The model under review builds one solid part; all positions refer to its coordinate system, in mm. A direction names the side the tool comes from. Coordinates: 2 decimals unless noted, no trailing zeros. Order: outer loops, then holes, each group sorted by start corner. A loop starts at its lowest first (then second) coordinate and runs counter-clockwise, first axis right, second up. Notation, with made-up numbers: (40.5, 25) -> (75.5, 25) arc R15 ccw to (75.5, 31) -> close; hole circle Ø2 at (38.5, 7.5). An arc over 180 degrees is marked (long way). Answer as CSV lines item,"result". Start each with the question number.
from build123d import *
from OCP.BRepFilletAPI import BRepFilletAPI_MakeFillet

# Parameters (mm, degrees)
CROQUIS2_W                 = 40
CROQUIS2_H                 = 15
SALIENTE_EXTRUIR1_DEPTH    = 65.5
REDONDEO1_R                = 1
CORTAR_EXTRUIR1_DEPTH      = 40
CORTAR_EXTRUIR4_DEPTH      = 1
CORTAR_EXTRUIR4_DEPTH_BACK = 10
CROQUIS9_W                 = 6
CROQUIS9_H                 = 15
CROQUIS10_W                = 6
CROQUIS10_H                = 15
CORTAR_EXTRUIR5_DEPTH      = 10
CROQUIS7_R                 = 2
CORTAR_EXTRUIR6_DEPTH      = 40
CROQUIS14_W                = 40.000001659
CROQUIS14_H                = 60.5
CORTAR_EXTRUIR9_DEPTH      = 2.6
REDONDEO5_R1               = 5
REDONDEO5_R2               = 1
CROQUIS16_W                = 32
CROQUIS16_H                = 4
CORTAR_EXTRUIR10_DEPTH     = 2.5


with BuildPart() as part:
    # Croquis2 → Saliente-Extruir1 (new body)
    with BuildSketch(Plane.XY):
        Rectangle(CROQUIS2_W, CROQUIS2_H)
    extrude(amount=SALIENTE_EXTRUIR1_DEPTH)

    # Redondeo1
    redondeo1_edges = [part.edges().sort_by_distance(p)[0] for p in [
        (-20, 0, 65.5),
        (0, -7.5, 65.5),
        (20, 0, 65.5),
        (0, -7.5, 0),
        (-20, 0, 0),
        (0, 7.5, 0),
        (20, 0, 0),
        (0, 7.5, 65.5),
        (20, -7.5, 32.75),
        (-20, -7.5, 32.75),
        (-20, 7.5, 32.75),
        (20, 7.5, 32.75),
    ]]
    fillet(redondeo1_edges, radius=REDONDEO1_R)

    # Croquis6 → Cortar-Extruir1 (cut)
    with BuildSketch(Plane(origin=(20, 0, 0), x_dir=(0, 0, -1), z_dir=(1, 0, 0))):
        Polygon((-60.5, 7.5), (-60.5, 0), (-55.501553512, 0), (-10, 0), (-10, 5), (-10, 7.5), align=None)
    extrude(amount=-CORTAR_EXTRUIR1_DEPTH, mode=Mode.SUBTRACT)

    # Croquis9 → Cortar-Extruir4 (cut, two sides: drawn at the far end of the back side and taken through both)
    with BuildSketch(Plane(origin=(0, 0, 0), x_dir=(-1, 0, 0), z_dir=(0, 0, -1)).offset(-CORTAR_EXTRUIR4_DEPTH_BACK)):
        with Locations((-17, 0)):
            Rectangle(CROQUIS9_W, CROQUIS9_H)
    extrude(amount=CORTAR_EXTRUIR4_DEPTH + CORTAR_EXTRUIR4_DEPTH_BACK, mode=Mode.SUBTRACT)

    # Croquis10 → Cortar-Extruir5 (cut)
    with BuildSketch(Plane(origin=(0, 0, 0), x_dir=(-1, 0, 0), z_dir=(0, 0, -1))):
        with Locations((17, 0)):
            Rectangle(CROQUIS10_W, CROQUIS10_H)
    extrude(amount=-CORTAR_EXTRUIR5_DEPTH, mode=Mode.SUBTRACT)

    # Croquis7 → Cortar-Extruir6 (cut)
    with BuildSketch(Plane(origin=(20, 0, 0), x_dir=(0, 0, -1), z_dir=(1, 0, 0))):
        with Locations((-5, 0)):
            Circle(CROQUIS7_R)
    extrude(amount=-CORTAR_EXTRUIR6_DEPTH, mode=Mode.SUBTRACT)

    # Croquis14 → Cortar-Extruir9 (cut)
    with BuildSketch(Plane(origin=(0, 7.5, 0), x_dir=(1, 0, 0), z_dir=(0, 1, 0))):
        with Locations((8.3e-07, -30.25)):
            Rectangle(CROQUIS14_W, CROQUIS14_H)
    extrude(amount=-CORTAR_EXTRUIR9_DEPTH, mode=Mode.SUBTRACT)

    # Redondeo5: one fillet with a radius per group of edges: ONE call of the kernel's fillet builder (fillet() takes one radius for all edges)
    redondeo5_edges_1 = [part.edges().sort_by_distance(p)[0] for p in [
        (0, 4.9, 0),
    ]]
    redondeo5_edges_2 = [part.edges().sort_by_distance(p)[0] for p in [
        (0, 4.9, 10),
    ]]
    redondeo5 = BRepFilletAPI_MakeFillet(part.part.solid().wrapped)
    for e in redondeo5_edges_1:
        redondeo5.Add(REDONDEO5_R1, e.wrapped)
    for e in redondeo5_edges_2:
        redondeo5.Add(REDONDEO5_R2, e.wrapped)
    add(Compound.cast(redondeo5.Shape()), mode=Mode.REPLACE)

    # Croquis16 → Cortar-Extruir10 (cut)
    with BuildSketch(Plane(origin=(0, 0, 0), x_dir=(1, 0, 0), z_dir=(0, 1, 0))):
        with Locations((0, -36.35)):
            Rectangle(CROQUIS16_W, CROQUIS16_H)
    extrude(amount=-CORTAR_EXTRUIR10_DEPTH, mode=Mode.SUBTRACT)


solid = part.part
1) Consider section A-A (x = 0). Give the boundary of the cut face in (y, z), plus the area to 3 significant figures.
2) Mouldability with a two-part tool opening along X and no side actions: class faces 4 (the face through (0.2, -1.2, 6.6)), 5 (the face through (14, -3, 5)), 6 (the face through (-16, -1, 36)), 7 (the face through (0, -1, 34.35)) as released by +X, released by -X, zero draft, split by the parting line, or undercut.
3) Consider section B-B (y = 2.75). Give the boundary of the cut face in (x, z), plus the area to 3 significant figures.
4) Wall thickness on L1, parallel to Y at x = 4, z = 5; L2, parallel to Z at x = 0.5, y = -1; L3, parallel to X at y = 1.75, z = 8: over which ranges is each line inside the solid? List them lowest first. Write a range as [from, to].
5) Consider section D-D (y = -5.5). Give the boundary of the cut face in (x, z).
6) Insertion check: pin 1 Ø8 at (x, y) = (4.5, 5.5) entering from -Z; pin 2 Ø8 at (y, z) = (-3.5, 5.5) entering from +X; pin 3 Ø3 at (x, z) = (2.5, 8) entering from +Y. Each pin has a flat end and moves straight along its axis. Give the tip position at first contact, or say it passes through.
7) Tool access review of faces 1 (the face through (0, 4.9, 7)), 2 (the face through (0, -1, 38.35)), 3 (the face through (0, 0, 41)): name each direction out of +Z, -Z, +X, -X, +Y, -Y from which nothing blocks a thin tool from reaching the whole face with its end or side.
8) Consider section C-C (z = 51). Give the boundary of the cut face in (x, y), plus the area to 3 significant figures.
Result:
1,outline,"(-7.5, 1) arc R1 ccw to (-6.5, 0) -> (-0.1, 0) arc R5 ccw to (4.9, 5) -> (4.9, 9) arc R1 ccw to (3.9, 10) -> (0, 10) -> (0, 34.35) -> (-2.5, 34.35) -> (-2.5, 38.35) -> (0, 38.35) -> (0, 60.5) -> (7.5, 60.5) -> (7.5, 64.5) arc R1 ccw to (6.5, 65.5) -> (-6.5, 65.5) arc R1 ccw to (-7.5, 64.5) -> close; hole circle Ø4 at (0, 5)"
1,area,"549 mm2"
2,face 4,"zero draft"
2,face 5,"released by +X"
2,face 6,"undercut"
2,face 7,"undercut"
3,outline,"(-20, 60.5) -> (20, 60.5) -> (20, 64.5) arc R1 ccw to (19, 65.5) -> (-19, 65.5) arc R1 ccw to (-20, 64.5) -> close; (-14, 0.89) -> (14, 0.89) -> (14, 10) -> (-14, 10) -> close"
3,area,"455 mm2"
4,L1,"[-7.5, -2], [2, 4.9]"
4,L2,"[0, 3.27], [6.73, 34.35], [38.35, 65.5]"
4,L3,"[-14, 14]"
5,outline,"(-20, 10) -> (-14, 10) -> (-14, 0) -> (14, 0) -> (14, 10) -> (20, 10) -> (20, 64.5) arc R1 ccw to (19, 65.5) -> (-19, 65.5) arc R1 ccw to (-20, 64.5) -> close"
6,pin 1,"z = 0.26"
6,pin 2,"x = 14"
6,pin 3,"y = 4.9"
7,face 1,"-Z, +X, -X, +Y"
7,face 2,"+Y"
7,face 3,"+X, -X, +Y"
8,outline,"(-20, -6.5) arc R1 ccw to (-19, -7.5) -> (19, -7.5) arc R1 ccw to (20, -6.5) -> (20, 0) -> (-20, 0) -> close"
8,area,"300 mm2"
